```python
from build123d import *

# Parameters (mm, degrees)
SKETCH_W        = 200
SKETCH_H        = 110
PAD_DEPTH       = 50
SKETCH001_W     = 16
SKETCH001_H     = 9
POCKET_DEPTH    = 1.7
SKETCH002_W     = 12
SKETCH002_H     = 108.3
POCKET001_DEPTH = 27
SKETCH003_R     = 1.25
POCKET002_DEPTH = 10
SKETCH004_W     = 179.6
SKETCH004_H     = 46.6
POCKET003_DEPTH = 106.6
SKETCH005_W     = 5
SKETCH005_H     = 108.3
POCKET004_DEPTH = 40
CHAMFER_SIZE    = 4.99
SKETCH006_R     = 28.5
POCKET005_DEPTH = 5


with BuildPart() as part:
    # Sketch → Pad (new body)
    with BuildSketch(Plane.XY):
        with Locations((100, 55)):
            Rectangle(SKETCH_W, SKETCH_H)
    extrude(amount=PAD_DEPTH)

    # Sketch001 (on Face1 of Pad) → Pocket (cut)
    with BuildSketch(Plane.XZ):
        with Locations((93.5, 14.5)):
            Rectangle(SKETCH001_W, SKETCH001_H)
    extrude(amount=-POCKET_DEPTH, mode=Mode.SUBTRACT)

    # Sketch002 (on Face4 of Pocket) → Pocket001 (cut)
    with BuildSketch(Plane.XY.offset(50)):
        with Locations((194, 54.15)):
            Rectangle(SKETCH002_W, SKETCH002_H)
    extrude(amount=-POCKET001_DEPTH, mode=Mode.SUBTRACT)

    # Sketch003 (on Face2 of Pocket001) → Pocket002 (cut)
    with BuildSketch(Plane(origin=(0, 0, 0), x_dir=(1, 0, 0), z_dir=(0, 0, -1))):
        with Locations((12.5, -12.5)):
            Circle(SKETCH003_R)
        with Locations((12.5, -97.5)):
            Circle(SKETCH003_R)
        with Locations((138.5, -97.5)):
            Circle(SKETCH003_R)
        with Locations((138.5, -12.5)):
            Circle(SKETCH003_R)
    extrude(amount=-POCKET002_DEPTH, mode=Mode.SUBTRACT)

    # Sketch004 (on Face18 of Pocket002) → Pocket003 (cut)
    with BuildSketch(Plane.XZ.offset(-1.7)):
        with Locations((96.5, 25)):
            Rectangle(SKETCH004_W, SKETCH004_H)
    extrude(amount=-POCKET003_DEPTH, mode=Mode.SUBTRACT)

    # Sketch005 (on Face6 of Pocket003) → Pocket004 (cut)
    with BuildSketch(Plane.XY.offset(50)):
        with Locations((2.5, 54.15)):
            Rectangle(SKETCH005_W, SKETCH005_H)
    extrude(amount=-POCKET004_DEPTH, mode=Mode.SUBTRACT)

    # Chamfer
    chamfer_edges = [part.edges().sort_by_distance(p)[0] for p in [
        (0, 54.15, 10),
    ]]
    chamfer(chamfer_edges, length=CHAMFER_SIZE)

    # Sketch006 (on Face6 of Chamfer) → Pocket005 (cut)
    with BuildSketch(Plane.XY.offset(50)):
        with Locations((47, 70)):
            Circle(SKETCH006_R)
    extrude(amount=-POCKET005_DEPTH, mode=Mode.SUBTRACT)


solid = part.part
```
Source: CAD feature listing. Evaluate the final solid. Frame: model axes, mm. A direction names the side the tool comes from. Coordinates: 2 decimals unless noted, no trailing zeros. Write each loop counter-clockwise with the first axis right and the second up, starting at its lowest first coordinate (ties: lowest second). Pieces come first, ordered by that corner, then holes. Notation, with made-up numbers: (-39.75, -6) -> (13.25, -6) arc R26 cw to (13.25, 15) -> close; hole circle Ø5 at (-8.5, 45). An arc over 180 degrees is marked (long way). Return JSON: item names as keys, results as strings. Group by question number.
1) Ray query, line 1 along Y through (x, z) = (12.5, 0.55); line 2 along X through (y, z) = (12.5, 1.15); line 3 along X through (y, z) = (19, 19.5). Return the intervals inside material, ascending.
2) Set-up query: faces 4 (the face through (194, 108.3, 37)), 5 (the face through (95, 108.3, 25)), 6 (the face through (2.53, 53.39, 7.54)). Return all of +Z, -Z, +X, -X, +Y, -Y with unobstructed straight access to the full face (end or side cutting, diameter ignored); none if empty.
3) Section query A-A, the plane z = 28. Return loops of the section in (x, y), plus the area to 3 significant figures.
4) Section query B-B, the plane x = 47. Return loops of the section in (y, z).
5) Section query D-D, the plane x = 104. Return loops of the section in (y, z).
6) Mould query, pull axis Y, two halves, no side actions, for faces 1 (the face through (200, 54, 8)), 2 (the face through (99, 110, 25)), 3 (the face through (6.7, 54, 25)). Classes: +Y half, -Y half, draft (parallel to the pull), parting line (faces both ways), or undercut.
7) Contact query for flat-ended pins moving along their axis: P1, Ø4, axis at x = 1.5, z = 27.5, coming from the -Y side; P2, Ø14, axis at y = 44, z = 23.5, coming from the -X side; P3, Ø2, axis at y = 56, z = 36, coming from the +X side. Output: stop coordinate, or through.
From the geometry:
{
 "1": {"line 1": "0 to 11.25, 13.75 to 96.25, 98.75 to 110", "line 2": "0 to 11.25, 13.75 to 137.25, 139.75 to 200", "line 3": "5 to 6.7, 186.3 to 200"},
 "2": {"face 4": "+Z, +X, -Y", "face 5": "none", "face 6": "+Z, -X, -Y"},
 "3": {"outline": "(0, 108.3) -> (5, 108.3) -> (5, 0) -> (188, 0) -> (188, 108.3) -> (200, 108.3) -> (200, 110) -> (0, 110) -> close; hole (6.7, 1.7) -> (186.3, 1.7) -> (186.3, 108.3) -> (6.7, 108.3) -> close", "area": "1,010 mm²"},
 "4": {"outline": "(0, 0) -> (110, 0) -> (110, 50) -> (98.5, 50) -> (98.5, 48.3) -> (108.3, 48.3) -> (108.3, 1.7) -> (1.7, 1.7) -> (1.7, 48.3) -> (41.5, 48.3) -> (41.5, 50) -> (0, 50) -> close"},
 "5": {"outline": "(0, 0) -> (110, 0) -> (110, 50) -> (0, 50) -> close; hole (1.7, 1.7) -> (108.3, 1.7) -> (108.3, 48.3) -> (1.7, 48.3) -> close"},
 "6": {"face 1": "draft", "face 2": "+Y half", "face 3": "undercut"},
 "7": {"P1": "y = 108.3", "P2": "x = 5", "P3": "x = 188"}
}
